Check sheet for the modelled part. Datum: model origin and axes. Units: mm. Face numbers are marked on the shaded views. A direction names the side the tool comes from. Give positions to 0.01 mm unless a question says otherwise; leave off trailing zeros. Loops run counter-clockwise (first coordinate to the right, second up) from the corner with the lowest first, then second, coordinate; pieces in that order, holes last. Notation, with made-up numbers: (-6.75, 16.5) -> (-1.75, 16.5) arc R18 cw to (-1.75, 50.5) -> close; hole circle Ø7 at (-9, 58). An arc over 180 degrees is marked (long way). Write each question's results on one line, items separated by ' | '. Start each with the question number.
Item 1: Cross-section at D-D on x = 33. Enter the section's corners in (y, z), then the cut area to 3 significant figures.
Item 2: Mould release check, pull along X, two halves, no side actions. Record for the marked faces 1, 2 and 3: pulls with the +X half, pulls with the -X half, needs draft (parallel to the pull), parting line crosses it, or undercut.
Item 3: Cross-section at A-A on x = 0. Enter the section's corners in (y, z), then the cut area to 3 significant figures.
Item 4: Access from +Z, -Z, +X, -X, +Y, -Y to the whole of each face (thin tool, end or side, straight path). Record for the marked faces 4 and 5.
Item 5: Cross-section at C-C on z = 2. Enter the section's corners in (x, y).
Item 6: Cross-section at B-B on y = -13.75. State how many separate pieces and enclosed holes the cut face has, then the cut area to 3 significant figures.
Item 7: Gauge pin test, flat ends, axial feed: pin 1 Ø6 at (x, y) = (14.5, -14) entering from -Z; pin 2 Ø5 at (x, y) = (-17.5, -11) entering from -Z; pin 3 Ø12 at (x, y) = (64.5, -7.5) entering from +Z. Record the tip position at first contact, or that the pin passes through.
Item 8: Scan lines: line 1 along X through (y, z) = (-11.25, 9); line 2 along X through (y, z) = (-21.5, 11.5); line 3 along Z through (x, y) = (-13, -13). Record each from-to range of solid material in increasing order.
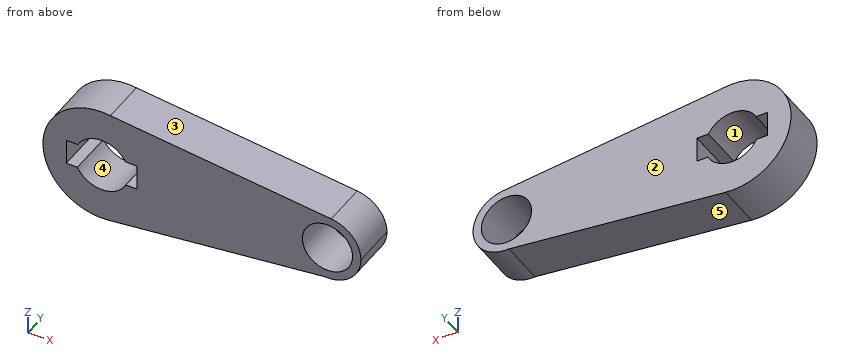
from build123d import *

# Parameters (mm, degrees)
F0_R     = 14.2875
F1_DEPTH = 25.4


with BuildPart() as f1:
    # F0 (on Front) → F1 (new body)
    with BuildSketch(Plane.XZ):
        with BuildLine():
            ThreePointArc((3.828865, -33.216132), (24.959907, -22.248027), (33.436083, 0))
            ThreePointArc((33.436083, 0), (25.336953, 21.817664), (4.963222, 33.065663))
            ThreePointArc((4.963222, 33.065663), (-33.431187, 0.572147), (3.828865, -33.216132))
        make_face()
        with BuildLine():
            ThreePointArc((-13.559361, 7.449858), (0, 15.471156), (13.559361, 7.449858))
            Line((13.559361, 7.449858), (20.06432, 7.449858))
            Line((20.06432, 7.449858), (20.06432, -6.998351))
            Line((20.06432, -6.998351), (13.797816, -6.998351))
            ThreePointArc((13.797816, -6.998351), (0, -15.471156), (-13.797816, -6.998351))
            Line((-13.797816, -6.998351), (-20.11976, -6.998351))
            Line((-20.11976, -6.998351), (-20.11976, 7.449858))
            Line((-20.11976, 7.449858), (-13.559361, 7.449858))
        make_face(mode=Mode.SUBTRACT)
        with BuildLine():
            ThreePointArc((4.963222, 33.065663), (25.336953, 21.817664), (33.436083, 0))
            ThreePointArc((33.436083, 0), (24.959907, -22.248027), (3.828865, -33.216132))
            Line((3.828865, -33.216132), (127.166579, -18.99884))
            ThreePointArc((127.166579, -18.99884), (109.593453, 1.762081), (130.690084, 18.930738))
            Line((130.690084, 18.930738), (4.963222, 33.065663))
        make_face()
        with BuildLine():
            ThreePointArc((147.611783, 0), (142.764717, 12.695637), (130.690084, 18.930738))
            ThreePointArc((130.690084, 18.930738), (109.593453, 1.762081), (127.166579, -18.99884))
            ThreePointArc((127.166579, -18.99884), (141.52951, -13.954948), (147.611783, 0))
        make_face()
        with Locations((128.561783, 0)):
            Circle(F0_R, mode=Mode.SUBTRACT)
    extrude(amount=F1_DEPTH)


solid = f1.part
Answer sheet:
1) outline: (-25.4, -29.85) -> (0, -29.85) -> (0, 29.91) -> (-25.4, 29.91) -> close | area: 1,520 mm²
2) face 1: undercut | face 2: needs draft | face 3: pulls with the +X half
3) outline: (-25.4, -33.44) -> (0, -33.44) -> (0, -15.47) -> (-25.4, -15.47) -> close; (-25.4, 15.47) -> (0, 15.47) -> (0, 33.44) -> (-25.4, 33.44) -> close | area: 913 mm²
4) face 4: +Y, -Y | face 5: -Z, +X, +Y, -Y
5) outline: (-33.38, -25.4) -> (-20.12, -25.4) -> (-20.12, 0) -> (-33.38, 0) -> close; (20.06, -25.4) -> (114.41, -25.4) -> (114.41, 0) -> (20.06, 0) -> close; (142.71, -25.4) -> (147.51, -25.4) -> (147.51, 0) -> (142.71, 0) -> close
6) separate pieces: 1 | enclosed holes: 2 | area: 7,550 mm²
7) pin 1: stops at z = -32.33 | pin 2: stops at z = -29.88 | pin 3: stops at z = 27.05
8) line 1: x = -32.2 to -12.58, 12.58 to 117.47, 139.66 to 145.35 | line 2: x = -31.4 to -10.35, 10.35 to 120.08, 137.04 to 143.75 | line 3: z = -30.81 to -8.39, 8.39 to 30.81
